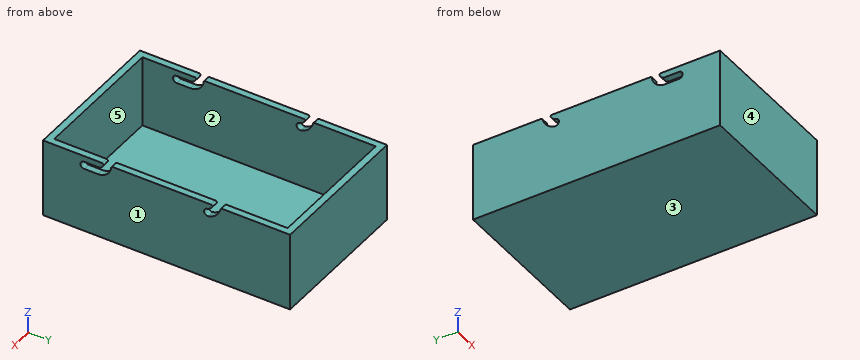
from build123d import *

# Parameters (mm, degrees)
ESQUISSE1_W             = 110
ESQUISSE1_H             = 180
ESQUISSE1_W_2           = 100
ESQUISSE1_H_2           = 170
BOSS_EXTRU_1_DEPTH      = 57
ESQUISSE2_W             = 110
ESQUISSE2_H             = 180
BOSS_EXTRU_2_DEPTH      = 5
ENL_V_MAT_EXTRU_1_DEPTH = 111
CONG_1_R                = 1


with BuildPart() as part:
    # Esquisse1 → Boss.-Extru.1 (new body)
    with BuildSketch(Plane.XY):
        with Locations((55, 90)):
            Rectangle(ESQUISSE1_W, ESQUISSE1_H)
        with Locations((55, 90)):
            Rectangle(ESQUISSE1_W_2, ESQUISSE1_H_2, mode=Mode.SUBTRACT)
    extrude(amount=BOSS_EXTRU_1_DEPTH)

    # Esquisse2 → Boss.-Extru.2 (add)
    with BuildSketch(Plane(origin=(0, 0, 0), x_dir=(-1, 0, 0), z_dir=(0, 0, -1))):
        with Locations((-55, 90)):
            Rectangle(ESQUISSE2_W, ESQUISSE2_H)
    extrude(amount=-BOSS_EXTRU_2_DEPTH)

    # Esquisse3 → Enlèv. mat.-Extru.1 (cut, through all)
    with BuildSketch(Plane.ZY):
        with BuildLine():
            ThreePointArc((52.62207614, 119.356014971), (54.199469032, 122.258730766), (57, 124.011144421))
            Line((57, 124.011144421), (57, 129.5))
            ThreePointArc((57, 129.5), (56.714535858, 129.484866891), (56.432271686, 129.439637203))
            ThreePointArc((56.432271686, 129.439637203), (50.642732019, 126.341305275), (47.37792386, 120.643985029))
            ThreePointArc((47.37792386, 120.643985029), (49.356014971, 117.37792386), (52.62207614, 119.356014971))
        make_face()
        with BuildLine():
            Line((57, 129.5), (57, 124.011144421))
            ThreePointArc((57, 124.011144421), (57.282178821, 124.092165775), (57.567728314, 124.160362797))
            ThreePointArc((57.567728314, 124.160362797), (59.684866891, 127.085464142), (57, 129.5))
        make_face()
        with BuildLine():
            ThreePointArc((47.3, 40), (50, 42.7), (52.7, 40))
            ThreePointArc((52.7, 40), (53.959440841, 43.040559159), (57, 44.3))
            Line((57, 44.3), (57, 49.7))
            ThreePointArc((57, 49.7), (50.141064222, 46.858935778), (47.3, 40))
        make_face()
        with BuildLine():
            Line((57, 49.7), (57, 44.3))
            ThreePointArc((57, 44.3), (59.7, 47), (57, 49.7))
        make_face()
        with BuildLine():
            ThreePointArc((47.3, 40), (50, 37.3), (52.7, 40))
            ThreePointArc((52.7, 40), (50, 42.7), (47.3, 40))
        make_face()
        with BuildLine():
            Line((47.3, 40), (47.3, 30))
            ThreePointArc((47.3, 30), (50, 27.3), (52.7, 30))
            Line((52.7, 30), (52.7, 40))
            ThreePointArc((52.7, 40), (50, 37.3), (47.3, 40))
        make_face()
    extrude(amount=-ENL_V_MAT_EXTRU_1_DEPTH, mode=Mode.SUBTRACT)

    # Congé1
    cong_1_edges = [part.edges().sort_by_distance(p)[0] for p in [
        (2.5, 49.7, 57),
        (107.5, 49.7, 57),
        (107.5, 44.3, 57),
        (2.5, 44.3, 57),
        (2.5, 124.011144421, 57),
        (2.5, 129.5, 57),
        (107.5, 124.011144421, 57),
        (107.5, 129.5, 57),
    ]]
    fillet(cong_1_edges, radius=CONG_1_R)


solid = part.part
Work out the finished part from the listing and answer in its coordinate system (mm). Face numbers are marked on the shaded views. A direction names the side the tool comes from. Coordinates: 2 decimals unless noted, no trailing zeros. Loops run counter-clockwise (first coordinate to the right, second up) from the corner with the lowest first, then second, coordinate; pieces in that order, holes last. Notation, with made-up numbers: M 47.5,77.25 L 105.5,77.25 A12 cw 105.5,95.25 Z; hole C 28,78.25 d10. An arc over 180 degrees is marked long. Answer in a Markdown table with one row per item. Add a question column.
1. The mould has two halves that part along X. Classify the marked faces 1, 2 and 3: pulls with the +X half, pulls with the -X half, needs draft (parallel to the pull), parting line crosses it, or undercut.
2. Find section A-A, the plane z = 50. Write down the section's boundary in (x, y).
3. Find section D-D, the plane z = 42. Write down the section's boundary in (x, y), then the cut area to 3 significant figures.
4. Find section C-C, the plane y = 149. Write down the section's boundary in (x, z).
5. A tool of negligible diameter and unlimited length cuts with its end or side. For the marked faces 4 and 5, from which of +Z, -Z, +X, -X, +Y, -Y can it reach the whole face along a straight path? Write none if from no direction.
6. Consider L1, parallel to X at y = 17, z = 38; L2, parallel to Y at x = 38.5, z = 10; L3, parallel to Z at x = 19, y = 28. Determine where each line is inside the solid, lowest interval first.
7. Find section B-B, the plane x = 8. Write down the section's boundary in (y, z), then the cut area to 3 significant figures.
Reported:
| question | item | result |
|---|---|---|
| 1 | face 1 | pulls with the +X half |
| 1 | face 2 | undercut |
| 1 | face 3 | needs draft |
| 2 | outline | M 0,0 L 110,0 L 110,27.3 L 105,27.3 L 105,5 L 5,5 L 5,27.3 L 0,27.3 Z; M 0,46.71 L 5,46.71 L 5,117.3 L 0,117.3 Z; M 0,125.67 L 5,125.67 L 5,175 L 105,175 L 105,125.67 L 110,125.67 L 110,180 L 0,180 Z; M 105,46.71 L 110,46.71 L 110,117.3 L 105,117.3 Z |
| 3 | outline | M 0,0 L 110,0 L 110,180 L 0,180 Z; hole M 5,5 L 105,5 L 105,175 L 5,175 Z |
| 3 | area | 2,800 mm^2 |
| 4 | outline | M 0,0 L 110,0 L 110,57 L 105,57 L 105,5 L 5,5 L 5,57 L 0,57 Z |
| 5 | face 4 | +Z, -Z, +X, -X, -Y |
| 5 | face 5 | +Z |
| 6 | L1 | x = 0 to 5, 105 to 110 |
| 6 | L2 | y = 0 to 5, 175 to 180 |
| 6 | L3 | z = 0 to 5 |
| 7 | outline | M 0,0 L 180,0 L 180,57 L 175,57 L 175,5 L 5,5 L 5,57 L 0,57 Z |
| 7 | area | 1,420 mm^2 |
